Check sheet for the modelled part. Datum: model origin and axes. Units: mm. A direction names the side the tool comes from. Round coordinates to 2 decimals unless told otherwise and drop trailing zeros. Loops run counter-clockwise (first coordinate to the right, second up) from the corner with the lowest first, then second, coordinate; pieces in that order, holes last. Notation, with made-up numbers: (42.25, 49) -> (98.25, 49) arc R22 cw to (98.25, 80) -> close; hole circle Ø5 at (-0.75, 16.5). An arc over 180 degrees is marked (long way). Use one line per item in the form item = value. Start each with the question number.
(1) Go/stop test with flat-tipped pins: pin 1 (3 mm diameter, centred on x = 5, y = 20, fed in from -Z); pin 2 (5 mm diameter, centred on y = 20.5, z = -10.5, fed in from -X); pin 3 (4.5 mm diameter, centred on x = -1, z = -14, fed in from +Y); pin 4 (5 mm diameter, centred on x = -8.5, y = 21.5, fed in from +Z). Record where each tip stops, or that it passes through.
(2) Sectioned sample at C-C (y = 41.75). Record the cut outline in (x, z).
(3) Material ranges on probe 1 along X at (y, z) = (12.5, -0.5); probe 2 along X at (y, z) = (13, 6); probe 3 along Z at (x, y) = (3.5, 15), recorded low to high. Write a range as [from, to].
(4) Sectioned sample at B-B (z = -4). Record the cut outline in (x, y).
(5) Sectioned sample at D-D (x = -8). Record the cut outline in (y, z), and give its area (3 significant figures).
(6) Set-up check for faces 1 (the flat face through (-11.5, 41, -13)), 2 (the flat face through (-7, 0, 16)): record each of +Z, -Z, +X, -X, +Y, -Y from which the full face is reachable in a straight line by a thin tool's end or side.
(7) Draft check along X on faces 3 (the flat face through (0.1, 44, 17.3)), 4 (the cylindrical face through (5.407, 21.692, 17.169)), 5 (the cylindrical face through (0.16, 40.51, 17.47)). Enter one of: released by +X, released by -X, zero draft, split by the parting line, or undercut.
(8) Sectioned sample at A-A (x = 0). Record the cut outline in (y, z).
from build123d import *

# Parameters (mm, degrees)
SKETCH1_R           = 18
BOSS_EXTRUDE1_DEPTH = 44
SKETCH3_R           = 17
CUT_EXTRUDE2_DEPTH  = 51.833060109
SKETCH11_W          = 23
SKETCH11_H          = 15.641557415
CUT_EXTRUDE4_DEPTH  = 7
SKETCH13_R          = 1.25
CUT_EXTRUDE5_DEPTH  = 20
CIRPATTERN1_COUNT   = 3


with BuildPart() as part:
    # Sketch1 → Boss-Extrude1 (new body)
    with BuildSketch(Plane(origin=(0, 0, 0), x_dir=(1, 0, 0), z_dir=(0, 1, 0))):
        with Locations(Location((0, 0, 0), (0, 0, 270))):
            Circle(SKETCH1_R)
    extrude(amount=BOSS_EXTRUDE1_DEPTH)

    # Sketch3 → Cut-Extrude2 (cut, through all)
    with BuildSketch(Plane(origin=(0, 44, 0), x_dir=(1, 0, 0), z_dir=(0, 1, 0))):
        with Locations(Location((0, 0, 0), (0, 0, 270))):
            Circle(SKETCH3_R)
    extrude(amount=-CUT_EXTRUDE2_DEPTH, mode=Mode.SUBTRACT)

    # Sketch11 → Cut-Extrude4 (cut)
    with BuildSketch(Plane(origin=(0, 44, 0), x_dir=(1, 0, 0), z_dir=(0, 1, 0))):
        with Locations((0, 14.057671998)):
            Rectangle(SKETCH11_W, SKETCH11_H)
    extrude(amount=-CUT_EXTRUDE4_DEPTH, mode=Mode.SUBTRACT)

    # Sketch13 → Cut-Extrude5 (cut)
    with BuildSketch(Plane.XY):
        with Locations(Location((0, 41.75, 0), (0, 0, 180))):
            Circle(SKETCH13_R)
    cut_extrude5 = extrude(amount=CUT_EXTRUDE5_DEPTH, mode=Mode.SUBTRACT)

    # CirPattern1: Cut-Extrude5 ×3 about axis
    cirpattern1_axis = Axis((0, 0, 0), (0, 1, 0))
    for i in range(1, CIRPATTERN1_COUNT):
        add(cut_extrude5.rotate(cirpattern1_axis, i * 360 / CIRPATTERN1_COUNT), mode=Mode.SUBTRACT)


solid = part.part
Checks:
q1.pin_1 = -17.66
q1.pin_2 = -16.12
q1.pin_3 = through
q1.pin_4 = 16.97
q2.outline = (-16.18, -7.9) -> (-15.31, -7.39) arc R17 cw to (-1.25, 16.95) -> (-1.25, 17.96) arc R18 ccw to start; (-14.93, -10.06) arc R18 ccw to (-11.5, -13.85) -> (-11.5, -12.52) arc R17 cw to (-14.06, -9.56) -> close; (1.25, 16.95) arc R17 cw to (15.31, -7.39) -> (16.18, -7.9) arc R18 ccw to (1.25, 17.96) -> close; (11.5, -13.85) arc R18 ccw to (14.93, -10.06) -> (14.06, -9.56) arc R17 cw to (11.5, -12.52) -> close
q3.probe_1 = [-17.99, -16.99], [16.99, 17.99]
q3.probe_2 = [-16.97, -15.91], [15.91, 16.97]
q3.probe_3 = [-17.66, -16.64], [16.64, 17.66]
q4.outline = (-17.55, 0) -> (-16.52, 0) -> (-16.52, 44) -> (-17.55, 44) -> close; (16.52, 0) -> (17.55, 0) -> (17.55, 44) -> (16.52, 44) -> close
q5.outline = (0, -16.12) -> (37, -16.12) -> (37, -15) -> (0, -15) -> close; (0, 15) -> (44, 15) -> (44, 16.12) -> (0, 16.12) -> close
q5.area = 91.1 mm2
q6.face_1 = -Z, +Y
q6.face_2 = +Z, -Z, +X, -X, -Y
q7.face_3 = zero draft
q7.face_4 = split by the parting line
q7.face_5 = undercut
q8.outline = (0, -18) -> (37, -18) -> (37, -17) -> (0, -17) -> close; (0, 17) -> (40.5, 17) -> (40.5, 18) -> (0, 18) -> close; (43, 17) -> (44, 17) -> (44, 18) -> (43, 18) -> close
